Part model, mm, in its own coordinate system. Round coordinates to 2 decimals unless told otherwise and drop trailing zeros. Loops run counter-clockwise (first coordinate to the right, second up) from the corner with the lowest first, then second, coordinate; pieces in that order, holes last.
(1) Flat gauge pin, fed straight in: pin 1 (0.8 mm diameter, centred on y = 0.5, z = -41, fed in from +X). Where does the tip first touch, or does it go through?
(2) Cut at B-B on y = 0.4. Count the separate pieces of the cut face and the enclosed holes in it, then the cut area to 3 significant figures.
(3) Mould opens along X. For faces 1 (the face through (-67.014, 0.74, -0.87)), 2 (the face through (-39.97, 0.74, -38.75)), 3 (the face through (50.116, 0.74, 32.901)) say: +X half, -X half, draft (parallel to the pull), parting line (faces both ways), or undercut.
(4) Cut at C-C on z = -28. List the corners of the cut face in (x, y).
(5) Cut at A-A on x = -58. List the corners of the cut face in (y, z).
(6) Probe probe 1 along Z at (x, y) = (0, 1.05); probe 2 along Z at (x, y) = (41, 1.4); probe 3 along Z at (x, y) = (-6.5, 1.2). List the from-to ranges inside material, lowest first.
from build123d import *

# Parameters (mm, degrees)
SKETCH_1_R      = 1.5
EXTRUDE_1_DEPTH = 1.5


with BuildPart() as part:
    # Эскиз1 → Бобышка-Вытянуть1 (new body)
    with BuildSketch(Plane(origin=(0, 0, 0), x_dir=(1, 0, 0), z_dir=(0, 1, 0))):
        with BuildLine():
            Line((-55.237590769, 32.053388295), (-61.7059188, 32.053388295))
            add(Edge.make_bspline(
                [(-61.7059188, 32.053388295), (-62.052521275, 32.031778061), (-62.744091711, 31.865477519), (-63.629073773, 31.277665282), (-64.260833863, 30.4238638), (-64.461976453, 29.741355241), (-64.501017169, 29.396222514)],
                knots=[0, 0, 0, 0, 0.25, 0.5, 0.75, 1, 1, 1, 1], degree=3))
            ThreePointArc((-64.501017169, 29.396222514), (-67.014010182, 0.462468283), (-64.469471559, -28.468528779))
            add(Edge.make_bspline(
                [(-64.469471559, -28.468528779), (-64.409048461, -28.810456535), (-64.166033983, -29.478831911), (-63.482303299, -30.291913357), (-62.562853807, -30.823470466), (-61.861851099, -30.946611705), (-61.514440275, -30.946611705)],
                knots=[0, 0, 0, 0, 0.25, 0.5, 0.75, 1, 1, 1, 1], degree=3))
            Line((-61.514440275, -30.946611705), (-55.237590769, -30.946611705))
            ThreePointArc((-55.237590769, -30.946611705), (-50.641396691, -32.850417627), (-48.737590769, -37.446611705))
            Line((-48.737590769, -37.446611705), (-48.737590769, -42.6958694))
            add(Edge.make_bspline(
                [(-48.737590769, -42.6958694), (-48.71091302, -43.077168109), (-48.507739461, -43.837500854), (-47.799680152, -44.773477074), (-46.795875092, -45.377409673), (-46.015918692, -45.499416665), (-45.633251479, -45.485174585)],
                knots=[0, 0, 0, 0, 0.25, 0.5, 0.75, 1, 1, 1, 1], degree=3))
            ThreePointArc((-45.633251479, -45.485174585), (-0.237590768, -46.223055901), (45.158069943, -45.485174585))
            add(Edge.make_bspline(
                [(45.158069943, -45.485174585), (45.539941303, -45.499387045), (46.317416103, -45.378581331), (47.323432889, -44.774398344), (48.030926989, -43.840884512), (48.235672001, -43.078018207), (48.26240923, -42.69586945)],
                knots=[0, 0, 0, 0, 0.25, 0.5, 0.75, 1, 1, 1, 1], degree=3))
            Line((48.26240923, -42.69586945), (48.26240923, -37.446611743))
            ThreePointArc((48.26240923, -37.446611743), (50.166215153, -32.850417666), (54.76240923, -30.946611743))
            Line((54.76240923, -30.946611743), (61.230737262, -30.946611743))
            add(Edge.make_bspline(
                [(61.230737262, -30.946611743), (61.577339736, -30.925001509), (62.268910172, -30.758700967), (63.153892234, -30.17088873), (63.785652325, -29.317087248), (63.986794915, -28.634578689), (64.025835631, -28.289445963)],
                knots=[0, 0, 0, 0, 0.25, 0.5, 0.75, 1, 1, 1, 1], degree=3))
            ThreePointArc((64.025835631, -28.289445963), (66.538853426, 0.553388257), (64.025835631, 29.396222476))
            add(Edge.make_bspline(
                [(64.025835631, 29.396222476), (63.98680709, 29.741247568), (63.785855195, 30.423449895), (63.154045977, 31.277502704), (62.269456107, 31.865245071), (61.577474792, 32.031769602), (61.230737261, 32.053388257)],
                knots=[0, 0, 0, 0, 0.25, 0.5, 0.75, 1, 1, 1, 1], degree=3))
            Line((61.230737261, 32.053388257), (54.762409231, 32.053388257))
            ThreePointArc((54.762409231, 32.053388257), (50.166215153, 33.957194179), (48.262409231, 38.553388257))
            Line((48.262409231, 38.553388257), (48.262409231, 43.802645952))
            add(Edge.make_bspline(
                [(48.262409231, 43.802645952), (48.235731482, 44.18394466), (48.032557923, 44.944277406), (47.324498614, 45.880253626), (46.320693554, 46.484186224), (45.540737153, 46.606193217), (45.158069941, 46.591951137)],
                knots=[0, 0, 0, 0, 0.25, 0.5, 0.75, 1, 1, 1, 1], degree=3))
            ThreePointArc((45.158069941, 46.591951137), (-0.237590771, 47.329832452), (-45.633251482, 46.591951137))
            add(Edge.make_bspline(
                [(-45.633251482, 46.591951137), (-46.015122842, 46.606163597), (-46.792597641, 46.485357883), (-47.798614427, 45.881174896), (-48.506108527, 44.947661064), (-48.71085354, 44.184794759), (-48.737590769, 43.802646001)],
                knots=[0, 0, 0, 0, 0.25, 0.5, 0.75, 1, 1, 1, 1], degree=3))
            Line((-48.737590769, 43.802646001), (-48.737590769, 38.553388295))
            ThreePointArc((-48.737590769, 38.553388295), (-50.641396691, 33.957194217), (-55.237590769, 32.053388295))
        make_face()
        with Locations(Location((-41.237590769, 39.553388295, 0), (0, 0, 270))):
            Circle(SKETCH_1_R, mode=Mode.SUBTRACT)
        with Locations(Location((-0.237590769, 39.553388295, 0), (0, 0, 270))):
            Circle(SKETCH_1_R, mode=Mode.SUBTRACT)
        with Locations(Location((40.762409231, 39.553388295, 0), (0, 0, 270))):
            Circle(SKETCH_1_R, mode=Mode.SUBTRACT)
        with Locations(Location((-41.237590769, -38.446611705, 0), (0, 0, 270))):
            Circle(SKETCH_1_R, mode=Mode.SUBTRACT)
        with Locations(Location((-0.237590769, -38.446611705, 0), (0, 0, 270))):
            Circle(SKETCH_1_R, mode=Mode.SUBTRACT)
        with Locations(Location((40.762409231, -38.446611705, 0), (0, 0, 270))):
            Circle(SKETCH_1_R, mode=Mode.SUBTRACT)
    extrude(amount=EXTRUDE_1_DEPTH)


solid = part.part
Final values:
1. pin 1: stops at x = 48.26
2. separate pieces: 1
2. enclosed holes: 6
2. area: 11,200 mm2
3. face 1: -X half
3. face 2: undercut
3. face 3: +X half
4. outline: (-64.74, 0) - (64.26, 0) - (64.26, 1.5) - (-64.74, 1.5) - close
5. outline: (0, -32.05) - (1.5, -32.05) - (1.5, 30.95) - (0, 30.95) - close
6. probe 1: z = -47.33 to -41.03, -38.07 to 36.97, 39.93 to 46.22
6. probe 2: z = -46.72 to -41.03, -38.07 to 36.97, 39.93 to 45.61
6. probe 3: z = -47.32 to 46.21
